```python
from build123d import *

# Parameters (mm, degrees)
FASE1_SIZE                           = 0.5
FASE2_SIZE                           = 1.3
SCHNITT_LINEAR_AUSTRAGEN1_DEPTH      = 15.75
SCHNITT_LINEAR_AUSTRAGEN1_DEPTH_BACK = 15.75
SKIZZE4_OUTSIDE_W                    = 41.778
SKIZZE4_OUTSIDE_H                    = 41.778
SKIZZE4_OUTSIDE_W_2                  = 20
SKIZZE4_OUTSIDE_H_2                  = 17
SCHNITT_LINEAR_AUSTRAGEN2_DEPTH      = 0.5


with BuildPart() as part:
    # Skizze2 → Rotation1 (revolve)
    with BuildSketch(Plane(origin=(0, 0, 0), x_dir=(0, 0, -1), z_dir=(1, 0, 0))):
        Polygon((0, 14.75), (-1.5, 14.75), (-1.5, 13), (-2, 13), (-2, 7.15), (-8.2, 5), (-14.2, 5), (-14.2, 5.942548531), (-15, 5.942548531), (-15, 5), (-29.5, 5), (-29.5, 3.125), (-4.5, 3.125), (-4.5, 1.45), (-2, 1.45), (-2, 3.9), (0, 3.9), (0, 7.5), (0.5, 7.5), (0.5, 9.5), (0, 9.5), (0, 12.65), (-0.8, 12.65), (-0.8, 14.15), (0, 14.15), align=None)
    revolve(axis=Axis((0, 0, -10.606367747), (0, 0, 1)))

    # Fase1
    fase1_edges = [part.edges().sort_by_distance(p)[0] for p in [
        (0, -14.75, 1.5),
    ]]
    chamfer(fase1_edges, length=FASE1_SIZE)

    # Fase2
    fase2_edges = [part.edges().sort_by_distance(p)[0] for p in [
        (0, -3.125, 29.5),
    ]]
    chamfer(fase2_edges, length=FASE2_SIZE)

    # Skizze3 → Schnitt-Linear austragen1 (cut, two sides)
    with BuildSketch(Plane(origin=(0, 0, 0), x_dir=(1, 0, 0), z_dir=(0, 1, 0))) as schnitt_linear_austragen1_sk:
        with BuildLine():
            Line((1.85, -21.35), (1.85, -29.5))
            ThreePointArc((1.85, -29.5), (0, -31.35), (-1.85, -29.5))
            Line((-1.85, -29.5), (-1.85, -21.35))
            ThreePointArc((-1.85, -21.35), (0, -19.5), (1.85, -21.35))
        make_face()
    extrude(amount=SCHNITT_LINEAR_AUSTRAGEN1_DEPTH, mode=Mode.SUBTRACT)
    extrude(schnitt_linear_austragen1_sk.sketch, amount=-SCHNITT_LINEAR_AUSTRAGEN1_DEPTH_BACK, mode=Mode.SUBTRACT)

    # Skizze4 outside → Schnitt-Linear austragen2 (cut)
    with BuildSketch(Plane(origin=(0, 0, -0.5), x_dir=(-1, 0, 0), z_dir=(0, 0, -1))):
        Rectangle(SKIZZE4_OUTSIDE_W, SKIZZE4_OUTSIDE_H)
        Rectangle(SKIZZE4_OUTSIDE_W_2, SKIZZE4_OUTSIDE_H_2, mode=Mode.SUBTRACT)
    extrude(amount=-SCHNITT_LINEAR_AUSTRAGEN2_DEPTH, mode=Mode.SUBTRACT)


solid = part.part
```
Read the model definition and answer for the solid it produces. Units are mm, in the model's axes. A direction names the side the tool comes from. Coordinates: 2 decimals unless noted, no trailing zeros. Write each loop counter-clockwise with the first axis right and the second up, starting at its lowest first coordinate (ties: lowest second). Pieces come first, ordered by that corner, then holes. Notation, with made-up numbers: (65, 26.25) -> (96, 26.25) arc R14 ccw to (96, 51.25) -> close; hole circle Ø1 at (1.5, 63). An arc over 180 degrees is marked (long way). Answer as a JSON object with one key per item and string values.
Q1. Determine the mould class of faces 5 (the cylindrical face through (-0.14, -3.12, 16.18)), 6 (the conical face through (2.047, 4.936, 7.21)), 7 (the flat face through (0, 9, 0)) for opening direction Y: pulls with the +Y half, pulls with the -Y half, needs draft (parallel to the pull), parting line crosses it, or undercut.
The answers:
{"face 5": "undercut", "face 6": "parting line crosses it", "face 7": "needs draft"}
Q2. The part is cut by section A-A on z = 9. Give the vertices of the cut face in (x, y) (3 decimals), then the cut area to 3 significant figures.
The answers:
{"outline": "circle Ø10 at (0, 0); hole circle Ø6.25 at (0, 0)", "area": "47.9 mm2"}
Q3. The part is cut by section B-B on z = 20. Give the vertices of the cut face in (x, y) (3 decimals).
The answers:
{"outline": "(-1.265, -4.837) -> (-1.265, -2.858) arc R3.125 cw to (-1.265, 2.858) -> (-1.265, 4.837) arc R5 ccw to start; (1.265, -4.837) arc R5 ccw to (1.265, 4.837) -> (1.265, 2.858) arc R3.125 cw to (1.265, -2.858) -> close"}
Q4. Flat-ended cylindrical pins translate along their axes: pin 1 Ø7 at (x, y) = (0, 0) entering from +Z (3 decimals); pin 2 Ø4.5 at (x, y) = (-3, 0) entering from -Z; pin 3 Ø2.5 at (y, z) = (-3.5, 25.5) entering from -X; pin 4 Ø7 at (x, y) = (-1, -1) entering from +Z. Find the tip coordinate at first contact, or state that the pin passes through.
The answers:
{"pin 1": "stops at z = 28.575", "pin 2": "stops at z = 0", "pin 3": "stops at x = -4.47", "pin 4": "stops at z = 29.5"}
Q5. Consider line 1 (Y direction, x = 0, z = 0.6); line 2 (X direction, y = 0.25, z = 16); line 3 (Y direction, x = 0, z = -0.15). Determine where each line is inside the solid, lowest interval first. Write a range as [from, to].
The answers:
{"line 1": "y = [-14.75, -14.15], [-12.65, -3.9], [3.9, 12.65], [14.15, 14.75]", "line 2": "x = [-4.99, -3.11], [3.11, 4.99]", "line 3": "y = [-8.5, -7.5], [7.5, 8.5]"}
Q6. The part is cut by section C-C on z = 3.5. Give the vertices of the cut face in (x, y).
The answers:
{"outline": "circle Ø13.26 at (0, 0); hole circle Ø2.9 at (0, 0)"}
Q7. A tool of negligible diameter and unlimited length cuts with its end or side. For faces 1 (the flat face through (-1.85, -4, 25)), 2 (the cylindrical face through (-0.06, -1.45, 3.23)), 3 (the cylindrical face through (4.88, -1.08, 22.35)), 4 (the cylindrical face through (12.553, 6.529, 0.394)), from which of +Z, -Z, +X, -X, +Y, -Y can it reach the whole face along a straight path? Write none if from no direction.
The answers:
{"face 1": "+Z, +Y, -Y", "face 2": "+Z, -Z", "face 3": "+Z", "face 4": "-Z"}
